Could you check a few things on this model? Use its own coordinates, in mm. A direction names the side the tool comes from. Coordinates: 2 decimals unless noted, no trailing zeros. Write each loop counter-clockwise with the first axis right and the second up, starting at its lowest first coordinate (ties: lowest second). Pieces come first, ordered by that corner, then holes. Notation, with made-up numbers: (26.25, 40) - (34.25, 40) arc R22 cw to (34.25, 74) - close; hole circle Ø2 at (-27.5, 62.25). An arc over 180 degrees is marked (long way). Answer as a JSON object with one key per item and string values. Group by question number.
1) If we section it at B-B (x = 30): Write out the boundary of the cut face in (y, z).
2) We'd pull the mould along Z, two halves only. Please class faces 4 (the flat face through (6, 25, -4)), 5 (the flat face through (4, 42, 0)): released by +Z, released by -Z, zero draft, split by the parting line, or undercut.
3) If we section it at C-C (y = 23): Write out the boundary of the cut face in (x, z).
4) Please list where these lines run through material, in increasing order: line 1 along Z through (x, y) = (8, 34.5); line 2 along Y through (x, z) = (5, -4.5); line 3 along Y through (x, z) = (32, -4.5).
5) On a 3-axis mill with a long thin cutter (end or side, diameter ignored), from which of +Z, -Z, +X, -X, +Y, -Y can I reach the whole of each face in a straight line? I mean faces 1 (the flat face through (7, 24, 5)), 2 (the flat face through (3, 21, -17.5)), 3 (the flat face through (22, 3, 5)). Say none if no direction works.
6) Will these pins go through, and if not, where does the flat tip stop? pin 1 Ø4 at (y, z) = (23, 15) entering from -X; pin 2 Ø1.5 at (x, z) = (25, 2.5) entering from +Y; pin 3 Ø6 at (x, z) = (23, -8) entering from +Y; pin 4 Ø7.5 at (x, z) = (30.5, -12.5) entering from -Y.
7) If we section it at A-A (z = 0): Write out the boundary of the cut face in (x, y), plus the area to 3 significant figures.
8) If we section it at D-D (x = 12.5): Write out the boundary of the cut face in (y, z).
```python
from build123d import *

# Parameters (mm, degrees)
AUFSATZ_LINEAR_AUSTRAGEN1_DEPTH = 20.5
SKIZZE2_W                       = 33
SKIZZE2_H                       = 31
SCHNITT_LINEAR_AUSTRAGEN1_DEPTH = 35
SCHNITT_LINEAR_AUSTRAGEN2_DEPTH = 10
SCHNITT_LINEAR_AUSTRAGEN3_DEPTH = 10
SKIZZE5_W                       = 9.5
SKIZZE5_H                       = 36
SKIZZE5_W_2                     = 10
SKIZZE5_H_2                     = 28
SCHNITT_LINEAR_AUSTRAGEN4_DEPTH = 5.5
SKIZZE6_W                       = 28
SKIZZE6_H                       = 10
SKIZZE6_W_2                     = 36
SKIZZE6_H_2                     = 9.5
SCHNITT_LINEAR_AUSTRAGEN5_DEPTH = 5.5
AUFSATZ_LINEAR_AUSTRAGEN2_DEPTH = 9.5
AUFSATZ_LINEAR_AUSTRAGEN3_DEPTH = 9.5


with BuildPart() as part:
    # Skizze1 → Aufsatz-Linear austragen1 (new, symmetric)
    with BuildSketch(Plane.XY):
        Polygon((0, 0), (42, 0), (42, 7), (38, 7), (7, 38), (7, 42), (0, 42), align=None)
    extrude(amount=AUFSATZ_LINEAR_AUSTRAGEN1_DEPTH, both=True)

    # Skizze2 → Schnitt-Linear austragen1 (cut)
    with BuildSketch(Plane(origin=(42, 0, 0), x_dir=(0, 0, -1), z_dir=(1, 0, 0))):
        with Locations((0, 22.5)):
            Rectangle(SKIZZE2_W, SKIZZE2_H)
    extrude(amount=-SCHNITT_LINEAR_AUSTRAGEN1_DEPTH, mode=Mode.SUBTRACT)

    # Skizze3 → Schnitt-Linear austragen2 (cut)
    with BuildSketch(Plane(origin=(7, 0, 0), x_dir=(0, 0, -1), z_dir=(1, 0, 0))):
        with BuildLine():
            Line((-4, 19), (-4, 31))
            ThreePointArc((-4, 31), (0, 35), (4, 31))
            Line((4, 31), (4, 19))
            ThreePointArc((4, 19), (0, 15), (-4, 19))
        make_face()
    extrude(amount=-SCHNITT_LINEAR_AUSTRAGEN2_DEPTH, mode=Mode.SUBTRACT)

    # Skizze4 → Schnitt-Linear austragen3 (cut)
    with BuildSketch(Plane(origin=(0, 7, 0), x_dir=(1, 0, 0), z_dir=(0, 1, 0))):
        with BuildLine():
            Line((19, 4), (31, 4))
            ThreePointArc((31, 4), (35, 0), (31, -4))
            Line((31, -4), (19, -4))
            ThreePointArc((19, -4), (15, 0), (19, 4))
        make_face()
    extrude(amount=-SCHNITT_LINEAR_AUSTRAGEN3_DEPTH, mode=Mode.SUBTRACT)

    # Skizze5 → Schnitt-Linear austragen4 (cut)
    with BuildSketch(Plane.ZY):
        with Locations((12.75, 21)):
            Rectangle(SKIZZE5_W, SKIZZE5_H)
        with Locations((0, 22)):
            Rectangle(SKIZZE5_W_2, SKIZZE5_H_2)
        with Locations((-12.75, 21)):
            Rectangle(SKIZZE5_W, SKIZZE5_H)
    extrude(amount=-SCHNITT_LINEAR_AUSTRAGEN4_DEPTH, mode=Mode.SUBTRACT)

    # Skizze6 → Schnitt-Linear austragen5 (cut)
    with BuildSketch(Plane.XZ):
        with Locations((22, 0)):
            Rectangle(SKIZZE6_W, SKIZZE6_H)
        with Locations((21, 12.75)):
            Rectangle(SKIZZE6_W_2, SKIZZE6_H_2)
        with Locations((21, -12.75)):
            Rectangle(SKIZZE6_W_2, SKIZZE6_H_2)
    extrude(amount=-SCHNITT_LINEAR_AUSTRAGEN5_DEPTH, mode=Mode.SUBTRACT)

    # Skizze7 → Aufsatz-Linear austragen2 (add)
    with BuildSketch(Plane.XY.offset(8)):
        Polygon((3, 0.5), (8, 5.5), (5.5, 5.5), (5.5, 8), (0.5, 3), (3, 3), align=None)
    extrude(amount=AUFSATZ_LINEAR_AUSTRAGEN2_DEPTH)

    # Skizze8 → Aufsatz-Linear austragen3 (add)
    with BuildSketch(Plane.XY.offset(-17.5)):
        Polygon((3, 0.5), (8, 5.5), (5.5, 5.5), (5.5, 8), (0.5, 3), (3, 3), align=None)
    extrude(amount=AUFSATZ_LINEAR_AUSTRAGEN3_DEPTH)


solid = part.part
```
Here are the results:
{
 "1": {"outline": "(0, -20.5) - (15, -20.5) - (15, -16.5) - (7, -16.5) - (7, -4) - (5.5, -4) - (5.5, -5) - (0, -5) - (0, -8) - (5.5, -8) - (5.5, -17.5) - (0, -17.5) - close; (0, 5) - (5.5, 5) - (5.5, 4) - (7, 4) - (7, 16.5) - (15, 16.5) - (15, 20.5) - (0, 20.5) - (0, 17.5) - (5.5, 17.5) - (5.5, 8) - (0, 8) - close"},
 "2": {"face 4": "undercut", "face 5": "zero draft"},
 "3": {"outline": "(0, -20.5) - (22, -20.5) - (22, -16.5) - (7, -16.5) - (7, -4) - (5.5, -4) - (5.5, -5) - (0, -5) - (0, -8) - (5.5, -8) - (5.5, -17.5) - (0, -17.5) - close; (0, 5) - (5.5, 5) - (5.5, 4) - (7, 4) - (7, 16.5) - (22, 16.5) - (22, 20.5) - (0, 20.5) - (0, 17.5) - (5.5, 17.5) - (5.5, 8) - (0, 8) - close"},
 "4": {"line 1": "z = -20.5 to -16.5, 16.5 to 20.5", "line 2": "y = 0 to 8, 36 to 42", "line 3": "y = 5.5 to 7"},
 "5": {"face 1": "+X, +Y", "face 2": "-X", "face 3": "-Y"},
 "6": {"pin 1": "stops at x = 5.5", "pin 2": "passes through", "pin 3": "stops at y = 7", "pin 4": "stops at y = 5.5"},
 "7": {"outline": "(0, 0) - (8, 0) - (8, 5.5) - (15, 5.5) - (15, 7) - (7, 7) - (7, 15) - (5.5, 15) - (5.5, 8) - (0, 8) - close; (0, 36) - (5.5, 36) - (5.5, 35) - (7, 35) - (7, 42) - (0, 42) - close; (35, 5.5) - (36, 5.5) - (36, 0) - (42, 0) - (42, 7) - (35, 7) - close", "area": "171 mm²"},
 "8": {"outline": "(0, -20.5) - (32.5, -20.5) - (32.5, -16.5) - (7, -16.5) - (7, 16.5) - (32.5, 16.5) - (32.5, 20.5) - (0, 20.5) - (0, 17.5) - (5.5, 17.5) - (5.5, 8) - (0, 8) - (0, 5) - (5.5, 5) - (5.5, -5) - (0, -5) - (0, -8) - (5.5, -8) - (5.5, -17.5) - (0, -17.5) - close"}
}
